Solid Edge part; units mm, degrees
sketch "Sketch1" plane through (0, 0, 0) normal (0, 0, 1) x (1, 0, 0)
  line L0 (1.5, 0) -> (1.5, 6)
  line L1 (0, 6) -> (1.5, 6)
  line L2 (0, 0) -> (0, 6)
  line L3 (0, 0) -> (0, -3)
  line L4 (0, -3) -> (2.75, -3)
  line L5 (2.75, -3) -> (2.75, 0)
  line L6 (2.75, 0) -> (1.5, 0)
revolve "RevolvedProtrusion1" add sketch "Sketch1" angle 360 about axis through (0, 0, 0) along (0, 1, 0)
sketch "Sketch2" plane through (0, 0, 0) normal (1, 0, 0) x (0, 1, 0)
  line L0 (-3, 1.9365) -> (-1.7, 1.9365)
  line L1 (-0.582, 0) -> (-1.7, 1.9365)
  line L2 (-3, 0) -> (-0.582, 0)
  line L3 (-3, 0) -> (-3, 1.9365)
revolve "RevolvedCutout1" cut sketch "Sketch2" angle 360 about axis through (0, -4.5, 0) along (0, 1, 0)
sketch "Sketch3" plane through (0, -3, 0) normal (0, -1, 0) x (0, 0, 1)
  circle A0 centre (0, 0) radius 1.9365
  line L0 (-1.25, -0.7217) -> (0, -1.4434)
  line L1 (0, -1.4434) -> (1.25, -0.7217)
  line L2 (1.25, -0.7217) -> (1.25, 0.7217)
  line L3 (1.25, 0.7217) -> (0, 1.4434)
  line L4 (0, 1.4434) -> (-1.25, 0.7217)
  line L5 (-1.25, 0.7217) -> (-1.25, -0.7217)
extrude "Protrusion1" add sketch "Sketch3" against normal up to next
sketch "Sketch4" plane through (0, 0, 0) normal (0, 0, 1) x (1, 0, 0)
  line L0 (-1.4434, -3) -> (0, -3)
  line L1 (0, -3) -> (0, -2.6132)
  line L2 (0, -2.6132) -> (-1.4434, -3)
revolve "RevolvedCutout2" cut sketch "Sketch4" angle 360 about axis through (0, -4.5, 0) along (0, 1, 0)
fillet "Round1" radius 0.1 1 edges at (0, 0, -1.5)
fillet "Round2" radius 0.275 1 edges at (0, -3, -2.75)
chamfer "倒斜角_2" distance 0.2 angle 45 1 edges at (0, 6, -1.5)
cosmetic_thread "螺纹_3" thread depth 4.8
Can you work these out from the model? Positions are in its coordinate system, mm. A direction names the side the tool comes from. Give positions to 0.01 mm unless a question says otherwise; leave off trailing zeros. Order: outer loops, then holes, each group sorted by start corner. A loop starts at its lowest first (then second) coordinate and runs counter-clockwise, first axis right, second up. Notation, with made-up numbers: M -39,24 L -23,24 A6 cw -23,33 Z; hole C 57.25,-32.75 d5. An arc over 180 degrees is marked long. Write item = value, one per line. Start each with the question number.
Q1. We'd pull the mould along Z, two halves only. Please class faces 1 (the flat face through (-1.088, -2.164, -0.616)), 2 (the cylindrical face through (-1.5, 2.99, -0.07)), 3 (the flat face through (0, 6, 0)): pulls with the +Z half, pulls with the -Z half, needs draft (parallel to the pull), parting line crosses it, or undercut.
Q2. For faces 4 (the flat face through (1.088, -2.164, 0.616)), 5 (the cylindrical face through (-0.596, -1.343, 2.685)), 6 (the flat face through (2, 0, 0)), which set-ups out of +Z, -Z, +X, -X, +Y, -Y let a thin tool reach every point of the face, with its end or its side?
Q3. Will these pins go through, and if not, where does the flat tip stop? pin 1 Ø1 at (y, z) = (-0.5, 1.5) entering from +X; pin 2 Ø1.5 at (y, z) = (-2, -2) entering from +X.
Q4. Suppose I cut it at A-A (y = 2.75). Write out the boundary of the cut face in (x, z), plus the area to 3 significant figures.
Q5. Suppose I cut it at B-B (y = -1). Write out the boundary of the cut face in (x, z), plus the area to 3 significant figures.
Q6. I need wall thicknesses on probe 1 along Y at (x, z) = (1.7, -1.55); probe 2 along Y at (x, z) = (0.95, 0.3); probe 3 along Z at (x, y) = (-0.55, -0.75). Which ranges of each line are inside material? Lowest first, please. Write a range as [from, to].
Check result:
q1.face_1 = undercut
q1.face_2 = parting line crosses it
q1.face_3 = needs draft
q2.face_4 = -Y
q2.face_5 = +Y, -Y
q2.face_6 = +Y
q3.pin_1 = 2.56
q3.pin_2 = 2.45
q4.outline = C 0,0 d3
q4.area = 7.07 mm2
q5.outline = C 0,0 d5.5; hole C 0,0 d1.45
q5.area = 22.1 mm2
q6.probe_1 = [-3, 0]
q6.probe_2 = [-1.16, 6]
q6.probe_3 = [-2.69, 2.69]
